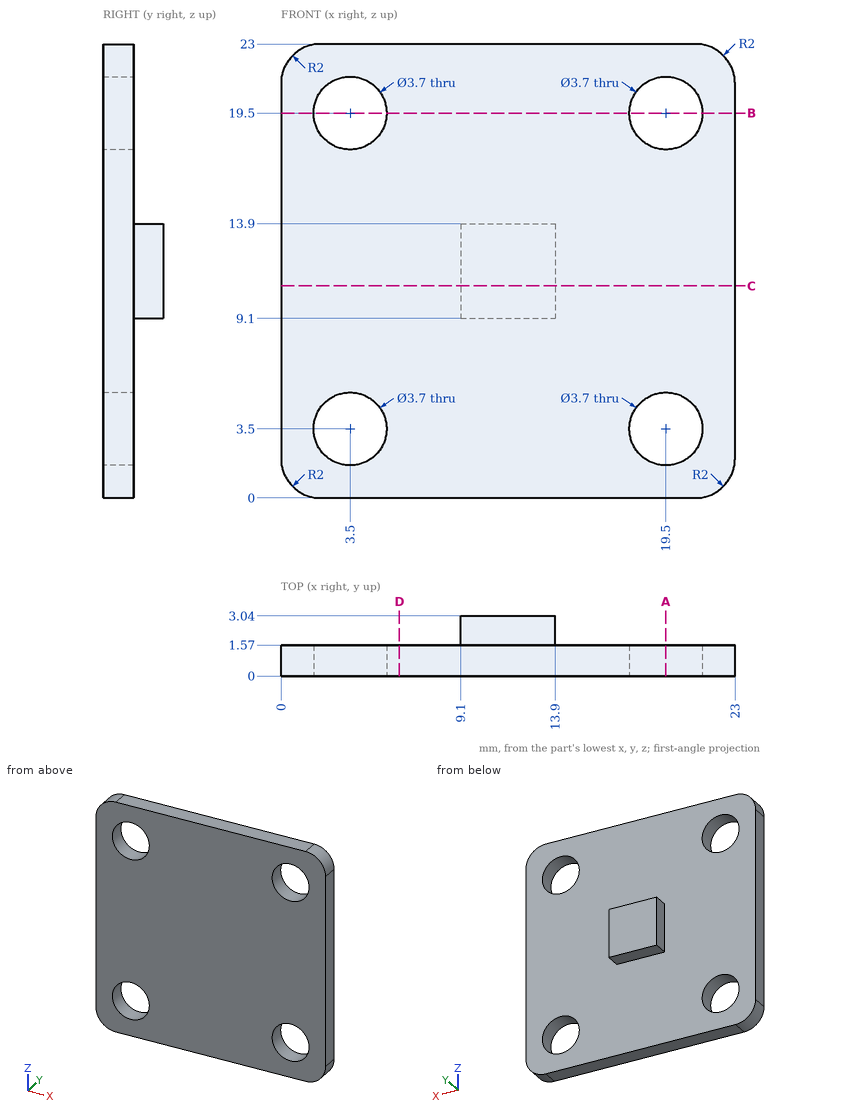
Job drawing, mm, ordinate dimensions from the low corner. One solid piece. Round coordinates to 2 decimals unless told otherwise and drop trailing zeros. Order: outer loops, then holes, each group sorted by start corner. A loop starts at its lowest first (then second) coordinate and runs counter-clockwise, first axis right, second up. Notation, with made-up numbers: (33.25, 74) - (76.25, 74) arc R5 cw to (76.25, 81) - close; hole circle Ø3 at (40.25, 81.5). An arc over 180 degrees is marked (long way). Use CSV: the item, a comma, the result in double quotes. Start each with the question number.
1) Pin check, flat tips, straight feed: pin 1 Ø5 at (x, z) = (3.5, 19.5) entering from +Y; pin 2 Ø1.2 at (y, z) = (2.5, 11.5) entering from -X; pin 3 Ø1.2 at (x, y) = (11, 2.5) entering from -Z. Stop position of each tip, or through.
2) Saw through at B-B (z = 19.5). List the corners of the cut face in (x, y), and give its area (3 significant figures).
3) Saw through at C-C (z = 10.75). List the corners of the cut face in (x, y), and give its area (3 significant figures).
4) Wall check: L1, parallel to X at y = 1, z = 19.5; L2, parallel to Z at x = 4, y = 0.7; L3, parallel to X at y = 0.2, z = 18.5. Give the ranges that are in metal, low to high. Write a range as [from, to].
5) Saw through at A-A (x = 19.5). List the corners of the cut face in (y, z).
6) Saw through at D-D (x = 6). List the corners of the cut face in (y, z).
Values follow:
1,pin 1,"stops at y = 1.57"
1,pin 2,"stops at x = 9.1"
1,pin 3,"stops at z = 9.1"
2,outline,"(0, 0) - (1.65, 0) - (1.65, 1.57) - (0, 1.57) - close; (5.35, 0) - (17.65, 0) - (17.65, 1.57) - (5.35, 1.57) - close; (21.35, 0) - (23, 0) - (23, 1.57) - (21.35, 1.57) - close"
2,area,"24.5 mm2"
3,outline,"(0, 0) - (23, 0) - (23, 1.57) - (13.9, 1.57) - (13.9, 3.04) - (9.1, 3.04) - (9.1, 1.57) - (0, 1.57) - close"
3,area,"43.2 mm2"
4,L1,"x = [0, 1.65], [5.35, 17.65], [21.35, 23]"
4,L2,"z = [0, 1.72], [5.28, 17.72], [21.28, 23]"
4,L3,"x = [0, 1.94], [5.06, 17.94], [21.06, 23]"
5,outline,"(0, 0) - (1.57, 0) - (1.57, 1.65) - (0, 1.65) - close; (0, 5.35) - (1.57, 5.35) - (1.57, 17.65) - (0, 17.65) - close; (0, 21.35) - (1.57, 21.35) - (1.57, 23) - (0, 23) - close"
6,outline,"(0, 0) - (1.57, 0) - (1.57, 23) - (0, 23) - close"
